Geometry check sheet. Reference: the model listing, model coordinates, mm. A direction names the side the tool comes from. Round coordinates to 2 decimals unless told otherwise and drop trailing zeros. Write each loop counter-clockwise with the first axis right and the second up, starting at its lowest first coordinate (ties: lowest second). Pieces come first, ordered by that corner, then holes. Notation, with made-up numbers: (21.25, 32.5) -> (28.25, 32.5) arc R23 cw to (28.25, 49.5) -> close; hole circle Ø10 at (59, 48). An arc over 180 degrees is marked (long way). Put each result on its own line as item: value. Start each with the question number.
from build123d import *

# Parameters (mm, degrees)
SKETCH1_R           = 6.5
SKETCH1_R_2         = 1
BOSS_EXTRUDE1_DEPTH = 7
SKETCH2_W           = 6.525565823
SKETCH2_H           = 1
CUT_EXTRUDE2_DEPTH  = 12.554220008
SKETCH3_R           = 1.25
CUT_EXTRUDE3_DEPTH  = 12.554220008
CUT_EXTRUDE5_START  = -2
CUT_EXTRUDE5_DEPTH  = 10.554220181
M2_TAPPED_HOLE2_D   = 1.6


with BuildPart() as part:
    # Sketch1 → Boss-Extrude1 (new body)
    with BuildSketch(Plane(origin=(0, 0, 0), x_dir=(0, 0, -1), z_dir=(1, 0, 0))):
        Circle(SKETCH1_R)
        Circle(SKETCH1_R_2, mode=Mode.SUBTRACT)
    extrude(amount=BOSS_EXTRUDE1_DEPTH)

    # Sketch2 → Cut-Extrude2 (cut, through all)
    with BuildSketch(Plane(origin=(0, 0, 0), x_dir=(0, 0, -1), z_dir=(1, 0, 0))):
        with Locations((3.262782911, 0)):
            Rectangle(SKETCH2_W, SKETCH2_H)
    extrude(amount=CUT_EXTRUDE2_DEPTH, mode=Mode.SUBTRACT)

    # Sketch3 → Cut-Extrude3 (cut, through all)
    with BuildSketch(Plane(origin=(0, 0, 0), x_dir=(1, 0, 0), z_dir=(0, 1, 0))):
        with Locations(Location((3.5, 3.5, 0), (0, 0, 270))):
            Circle(SKETCH3_R)
    extrude(amount=-CUT_EXTRUDE3_DEPTH, mode=Mode.SUBTRACT)

    # Sketch4 → Cut-Extrude5 (cut, through all)
    with BuildSketch(Plane(origin=(0, 0, 0), x_dir=(1, 0, 0), z_dir=(0, 1, 0)).offset(CUT_EXTRUDE5_START)):
        with BuildLine():
            Line((1.4, 3.5), (1.4, 9.014179598))
            Line((1.4, 9.014179598), (5.6, 9.014179598))
            Line((5.6, 9.014179598), (5.6, 3.5))
            ThreePointArc((5.6, 3.5), (3.5, 1.4), (1.4, 3.5))
        make_face()
    extrude(amount=-CUT_EXTRUDE5_DEPTH, mode=Mode.SUBTRACT)

    # M2 Tapped Hole2 (through all)
    with Locations(Plane(origin=(0, 0.5, 0), x_dir=(-1, 0, 0), z_dir=(0, -1, 0))):
        with Locations((-3.5, 3.5)):
            Hole(M2_TAPPED_HOLE2_D / 2)


solid = part.part
(1) Sectioned sample at D-D (x = 4.5). Record the cut outline in (y, z).
(2) Mould release check, pull along X, two halves, no side actions. Record for faces 6 (the flat face through (3, -0.5, -5)), 7 (the flat face through (7, -1.4, 0.1)), 8 (the flat face through (0, -1.4, 0.1)), 9 (the flat face through (4, -2, -5)): +X half, -X half, draft (parallel to the pull), parting line (faces both ways), or undercut.
(3) Sectioned sample at A-A (z = 0). Record the cut outline in (x, y), and give its area (3 significant figures).
(4) Set-up check for faces 1 (the flat face through (2.67, 0.5, -3.01)), 2 (the cylindrical face through (3, 0, 1)), 3 (the cylindrical face through (2.391, -1.24, -2.923)), 4 (the flat face through (1.4, -3, -5)), 5 (the cylindrical face through (3.33, 3.24, -2.72)): record each of +Z, -Z, +X, -X, +Y, -Y from which the full face is reachable in a straight line by a thin tool's end or side.
(5) Go/stop test with flat-tipped pins: pin 1 Ø4 at (x, z) = (4, -1.5) entering from +Y; pin 2 Ø1.5 at (x, z) = (5.5, -2) entering from +Y; pin 3 Ø1.8 at (x, z) = (3.5, -3.5) entering from +Y; pin 4 Ø1.8 at (y, z) = (0, 0) entering from -X. Record where each tip stops, or that it passes through.
(6) Sectioned sample at C-C (z = -4.5). Record the cut outline in (x, y).
(7) Material ranges on L1, parallel to X at y = -1.05, z = -3.5; L2, parallel to Y at x = 0.5, z = -3.5; L3, parallel to Z at x = 4.25, y = 0, recorded low to high. Write a range as from..to.
(8) Sectioned sample at B-B (x = 3.25). Record the cut outline in (y, z), and give its area (3 significant figures).
Found:
1. outline: (-6.29, -1.65) -> (-2, -1.65) -> (-2, -2.75) -> (-0.5, -2.75) -> (-0.5, -0.87) arc R1 cw (long way) to (0.5, -0.87) -> (0.5, -6.48) arc R6.5 ccw (long way) to start; (-2, -6.18) arc R6.5 ccw to (-0.5, -6.48) -> (-0.5, -4.25) -> (-2, -4.25) -> close
2. face 6: draft
2. face 7: +X half
2. face 8: -X half
2. face 9: undercut
3. outline: (0, -6.5) -> (7, -6.5) -> (7, -1) -> (0, -1) -> close; (0, 1) -> (7, 1) -> (7, 6.5) -> (0, 6.5) -> close
3. area: 77.0 mm2
4. face 1: -Z, +X, -X
4. face 2: +X, -X
4. face 3: -Y
4. face 4: -Z, -Y
4. face 5: +Y, -Y
5. pin 1: y = 6.5
5. pin 2: y = 6.38
5. pin 3: y = 5.96
5. pin 4: through
6. outline: (0, -4.69) -> (1.4, -4.69) -> (1.4, -2) -> (2.75, -2) -> (2.75, -0.5) -> (0, -0.5) -> close; (0, 0.5) -> (7, 0.5) -> (7, 4.69) -> (0, 4.69) -> close; (4.25, -2) -> (5.6, -2) -> (5.6, -4.69) -> (7, -4.69) -> (7, -0.5) -> (4.25, -0.5) -> close
7. L1: 0..2.25, 4.75..7
7. L2: -5.48..-0.5, 0.5..5.48
7. L3: 1..6.5
8. outline: (-6.34, -1.41) -> (-2, -1.41) -> (-2, -2.28) -> (-0.5, -2.28) -> (-0.5, -0.87) arc R1 cw (long way) to (0.5, -0.87) -> (0.5, -2.74) -> (5.89, -2.74) arc R6.5 ccw (long way) to start; (-2, -6.18) arc R6.5 ccw to (-0.5, -6.48) -> (-0.5, -4.72) -> (-2, -4.72) -> close; (0.5, -6.48) arc R6.5 ccw to (4.91, -4.26) -> (0.5, -4.26) -> close
8. area: 98.8 mm2
